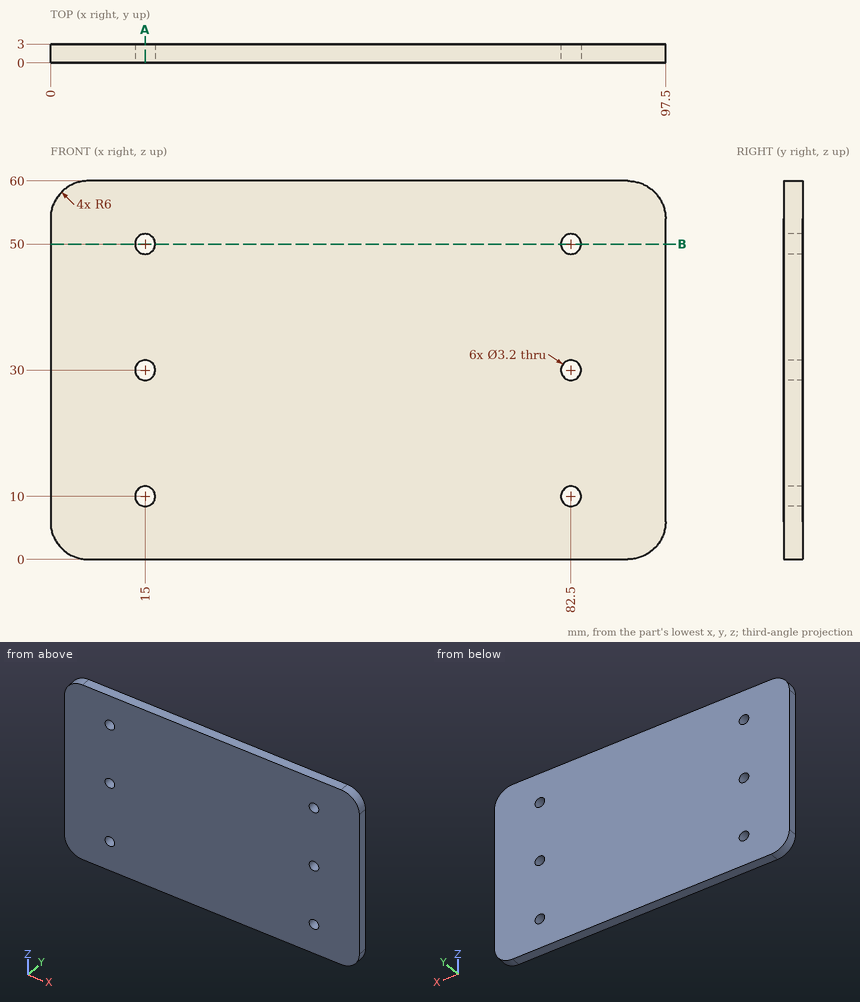
The drawing under review shows one solid part. Ordinate dimensions are in mm from its lowest x, y, z. Give positions to 0.01 mm unless a question says otherwise; leave off trailing zeros. Order: outer loops, then holes, each group sorted by start corner. A loop starts at its lowest first (then second) coordinate and runs counter-clockwise, first axis right, second up. Notation, with made-up numbers: (82.5, 62) - (129.5, 62) arc R23 ccw to (129.5, 80) - close; hole circle Ø3 at (5.5, 1.25). An arc over 180 degrees is marked (long way). Answer as a JSON object with one key per item and string values. Group by question number.
Item 1: Take a section at B-B on z = 50. Give the boundary of the cut face in (x, y), and give its area (3 significant figures).
Item 2: Wall thickness on line 1 along X through (y, z) = (0.7, 50); line 2 along Z through (x, y) = (82.5, 2.05); line 3 along Z through (x, y) = (82, 2.55): over which ranges is each line inside the solid? List them lowest first.
Item 3: Take a section at A-A on x = 15. Give the boundary of the cut face in (y, z), and give its area (3 significant figures).
Item 4: Clearance check with flat-ended pins moving along their axes: pin 1 Ø3.5 at (x, z) = (82.5, 10) entering from +Y; pin 2 Ø3 at (x, z) = (82.5, 30) entering from +Y. State where each tip first meets the part, or that it passes through.
Reported:
{
 "1": {"outline": "(0, 0) - (13.4, 0) - (13.4, 3) - (0, 3) - close; (16.6, 0) - (80.9, 0) - (80.9, 3) - (16.6, 3) - close; (84.1, 0) - (97.5, 0) - (97.5, 3) - (84.1, 3) - close", "area": "273 mm^2"},
 "2": {"line 1": "0 to 13.4, 16.6 to 80.9, 84.1 to 97.5", "line 2": "0 to 8.4, 11.6 to 28.4, 31.6 to 48.4, 51.6 to 60", "line 3": "0 to 8.48, 11.52 to 28.48, 31.52 to 48.48, 51.52 to 60"},
 "3": {"outline": "(0, 0) - (3, 0) - (3, 8.4) - (0, 8.4) - close; (0, 11.6) - (3, 11.6) - (3, 28.4) - (0, 28.4) - close; (0, 31.6) - (3, 31.6) - (3, 48.4) - (0, 48.4) - close; (0, 51.6) - (3, 51.6) - (3, 60) - (0, 60) - close", "area": "151 mm^2"},
 "4": {"pin 1": "y = 3", "pin 2": "through"}
}
